CAD build for the part. Positions are in the model's coordinates, mm. A direction names the side the tool comes from. Coordinates: 2 decimals unless noted, no trailing zeros. Order: outer loops, then holes, each group sorted by start corner. A loop starts at its lowest first (then second) coordinate and runs counter-clockwise, first axis right, second up. Notation, with made-up numbers: M 16,44.25 L 28,44.25 A25 cw 28,60.25 Z; hole C -35.5,-23 d8. An arc over 180 degrees is marked long. Write item = value, one per line.
from build123d import *

# Parameters (mm, degrees)
F0_W     = 0.8
F0_H     = 9
F0_W_2   = 1.2
F0_H_2   = 14.8
F1_DEPTH = 1.2
F2_DEPTH = 1.6
F3_DEPTH = 4.8
F4_DEPTH = 1.6


with BuildPart() as f1:
    # F0 (on Top) → F1 (new body)
    with BuildSketch(Plane.XY):
        Polygon((9.289006, -7.4), (9.289006, 7.4), (3.447185, 7.4), (0.247185, 10.4), (-10.310994, 10.4), (-10.310994, 4.5), (-10.310994, -4.5), (-10.310994, -10.4), (0.247185, -10.4), (3.447185, -7.4), align=None)
        with Locations((-10.710994, 0)):
            Rectangle(F0_W, F0_H)
        Polygon((10.489006, -8.2), (10.489006, -7.4), (9.289006, -7.4), (3.447185, -7.4), (0.247185, -10.4), (-10.310994, -10.4), (-10.310994, -4.5), (-11.110994, -4.5), (-11.110994, -11.2), (0.563543, -11.2), (3.763543, -8.2), align=None)
        with Locations((9.889006, 0)):
            Rectangle(F0_W_2, F0_H_2)
        Polygon((10.489006, 8.2), (3.763543, 8.2), (0.563543, 11.2), (-11.110994, 11.2), (-11.110994, 4.5), (-10.310994, 4.5), (-10.310994, 10.4), (0.247185, 10.4), (3.447185, 7.4), (9.289006, 7.4), (10.489006, 7.4), align=None)
    extrude(amount=F1_DEPTH)

    # F0 (on Top) → F2 (join)
    with BuildSketch(Plane.XY):
        with Locations((-10.710994, 0)):
            Rectangle(F0_W, F0_H)
    extrude(amount=F2_DEPTH)

    # F0 (on Top) → F3 (join)
    with BuildSketch(Plane.XY):
        with Locations((9.889006, 0)):
            Rectangle(F0_W_2, F0_H_2)
    extrude(amount=F3_DEPTH)

    # F0 (on Top) → F4 (join)
    with BuildSketch(Plane.XY):
        Polygon((9.289006, -7.4), (9.289006, 7.4), (3.447185, 7.4), (0.247185, 10.4), (-10.310994, 10.4), (-10.310994, 4.5), (-10.310994, -4.5), (-10.310994, -10.4), (0.247185, -10.4), (3.447185, -7.4), align=None)
    extrude(amount=F4_DEPTH)


solid = f1.part
(1) Pin check, flat tips, straight feed: pin 1 Ø1.5 at (y, z) = (3, 3.5) entering from -X; pin 2 Ø2 at (x, y) = (0, -8) entering from +Z; pin 3 Ø1.1 at (x, z) = (5.5, 3) entering from -Y; pin 4 Ø1.5 at (x, y) = (2.5, -3) entering from -Z. Stop position of each tip, or through.
Evaluation:
pin_1 = 9.29
pin_2 = 1.6
pin_3 = through
pin_4 = 0
(2) Slice it at A-A, the plane x = -1. Write the cut outline in (y, z), then the cut area to 3 significant figures.
Evaluation:
outline = M -11.2,0 L 11.2,0 L 11.2,1.2 L 10.4,1.2 L 10.4,1.6 L -10.4,1.6 L -10.4,1.2 L -11.2,1.2 Z
area = 35.2 mm²
(3) Wall check: line 1 (Z direction, x = -2.75, y = 3.75); line 2 (X direction, y = 4.5, z = 2.35); line 3 (Y direction, x = 7.5, z = 0.9). Give the ranges that are in metal, low to high. Write a range as from..to.
Evaluation:
line_1 = 0..1.6
line_2 = 9.29..10.49
line_3 = -8.2..8.2
(4) Slice it at B-B, the plane y = 5. Write the cut outline in (x, z).
Evaluation:
outline = M -11.11,0 L 10.49,0 L 10.49,4.8 L 9.29,4.8 L 9.29,1.6 L -10.31,1.6 L -10.31,1.2 L -11.11,1.2 Z
(5) Slice it at D-D, the plane y = -4. Write the cut outline in (x, z), then the cut area to 3 significant figures.
Evaluation:
outline = M -11.11,0 L 10.49,0 L 10.49,4.8 L 9.29,4.8 L 9.29,1.6 L -11.11,1.6 Z
area = 38.4 mm²
(6) Tool access for faces 1 (the face through (-1, 0, 1.6)), 2 (the face through (10, -7.4, 2)), 3 (the face through (7, -8.2, 1)), 4 (the face through (10, 7.4, 2)): list every direction of +Z, -Z, +X, -X, +Y, -Y with a clear straight run to the whole face (end or side of a thin tool).
Evaluation:
face_1 = +Z, -X, +Y, -Y
face_2 = +Z, +X, -Y
face_3 = +Z, -Z, +X, -Y
face_4 = +Z, +X, +Y
(7) Slice it at C-C, the plane z = 1.95. Write the cut outline in (x, y).
Evaluation:
outline = M 9.29,-7.4 L 10.49,-7.4 L 10.49,7.4 L 9.29,7.4 Z
